```python
from build123d import *

# Parameters (mm, degrees)
EXTRUDE_1_DEPTH = 20


with BuildPart() as part:
    # 草圖1 → 填料-伸長1 (new body)
    with BuildSketch(Plane.XY):
        with BuildLine():
            Line((0, 0), (15, 0))
            Line((15, 0), (15, 5))
            ThreePointArc((15, 5), (16.464466094, 8.535533906), (20, 10))
            Line((20, 10), (30, 10))
            Line((30, 10), (30, 15))
            Line((30, 15), (15, 15))
            ThreePointArc((15, 15), (11.464466094, 16.464466094), (10, 20))
            Line((10, 20), (10, 25))
            Line((10, 25), (5, 25))
            Line((5, 25), (5, 20))
            Line((5, 20), (-5, 20))
            Line((-5, 20), (-5, 5))
            Line((-5, 5), (0, 5))
            Line((0, 5), (0, 0))
        make_face()
    extrude(amount=EXTRUDE_1_DEPTH)


solid = part.part
```
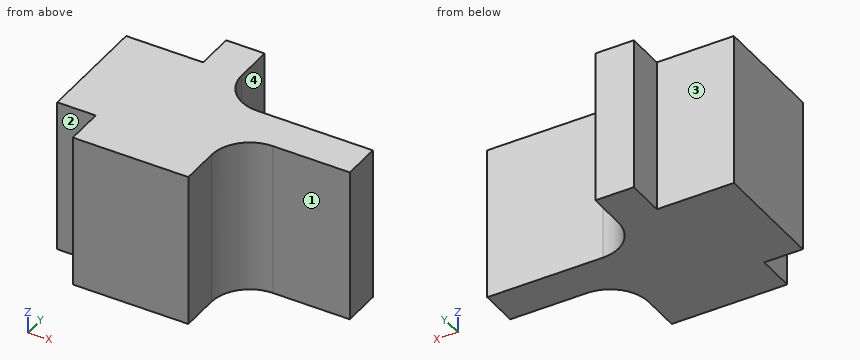
The listing builds one solid part. Answer for the finished solid, in the listing's coordinates (mm). Face numbers are marked on the shaded views. A direction names the side the tool comes from. Give positions to 0.01 mm unless a question says otherwise; leave off trailing zeros. Write each loop counter-clockwise with the first axis right and the second up, starting at its lowest first coordinate (ties: lowest second). Pieces come first, ordered by that corner, then holes. Notation, with made-up numbers: (87.25, 88) - (128.25, 88) arc R7 ccw to (128.25, 99) - close; hole circle Ø1 at (-20.75, -18). An arc over 180 degrees is marked (long way). Use one line per item in the form item = value. Start each with the question number.
1) Flat-ended cylindrical pins translate along their axes: pin 1 Ø1 at (y, z) = (21.5, 11) entering from +X; pin 2 Ø2.5 at (y, z) = (3, 6) entering from +X; pin 3 Ø1.5 at (x, z) = (-1.5, 7) entering from -Y. Find the tip coordinate at first contact, or state that the pin passes through.
2) Consider line 1 along X through (y, z) = (5.25, 15.75); line 2 along Y through (x, z) = (25, 11); line 3 along X through (y, z) = (19.75, 13.5). Determine where each line is inside the solid, lowest interval first. Write a range as from..to.
3) Find section B-B on x = 2. Determine the outline of the cut face in (y, z).
4) Find section C-C on y = 22. Determine the outline of the cut face in (x, z), plus the area to 3 significant figures.
5) A tool of negligible diameter and unlimited length cuts with its end or side. For the marked faces 1, 2, 3 and 4, from which of +Z, -Z, +X, -X, +Y, -Y can it reach the whole face along a straight path? Write none if from no direction.
6) Find section A-A on z = 11. Determine the outline of the cut face in (x, y).
Geometry results:
q1.pin_1 = 10
q1.pin_2 = 15
q1.pin_3 = 5
q2.line_1 = -5..15.01
q2.line_2 = 10..15
q2.line_3 = -5..10.01
q3.outline = (0, 0) - (20, 0) - (20, 20) - (0, 20) - close
q4.outline = (5, 0) - (10, 0) - (10, 20) - (5, 20) - close
q4.area = 100 mm2
q5.face_1 = +Z, -Z, +X, -Y
q5.face_2 = +Z, -Z, -X, -Y
q5.face_3 = +Z, -Z, -X, +Y
q5.face_4 = +Z, -Z, +X, +Y
q6.outline = (-5, 5) - (0, 5) - (0, 0) - (15, 0) - (15, 5) arc R5 cw to (20, 10) - (30, 10) - (30, 15) - (15, 15) arc R5 cw to (10, 20) - (10, 25) - (5, 25) - (5, 20) - (-5, 20) - close
